Source: three-view drawing plus pictorial views. Frame: mm from the lowest corner of the part. Give positions to 0.01 mm unless a question says otherwise; leave off trailing zeros. Order: outer loops, then holes, each group sorted by start corner. A loop starts at its lowest first (then second) coordinate and runs counter-clockwise, first axis right, second up.
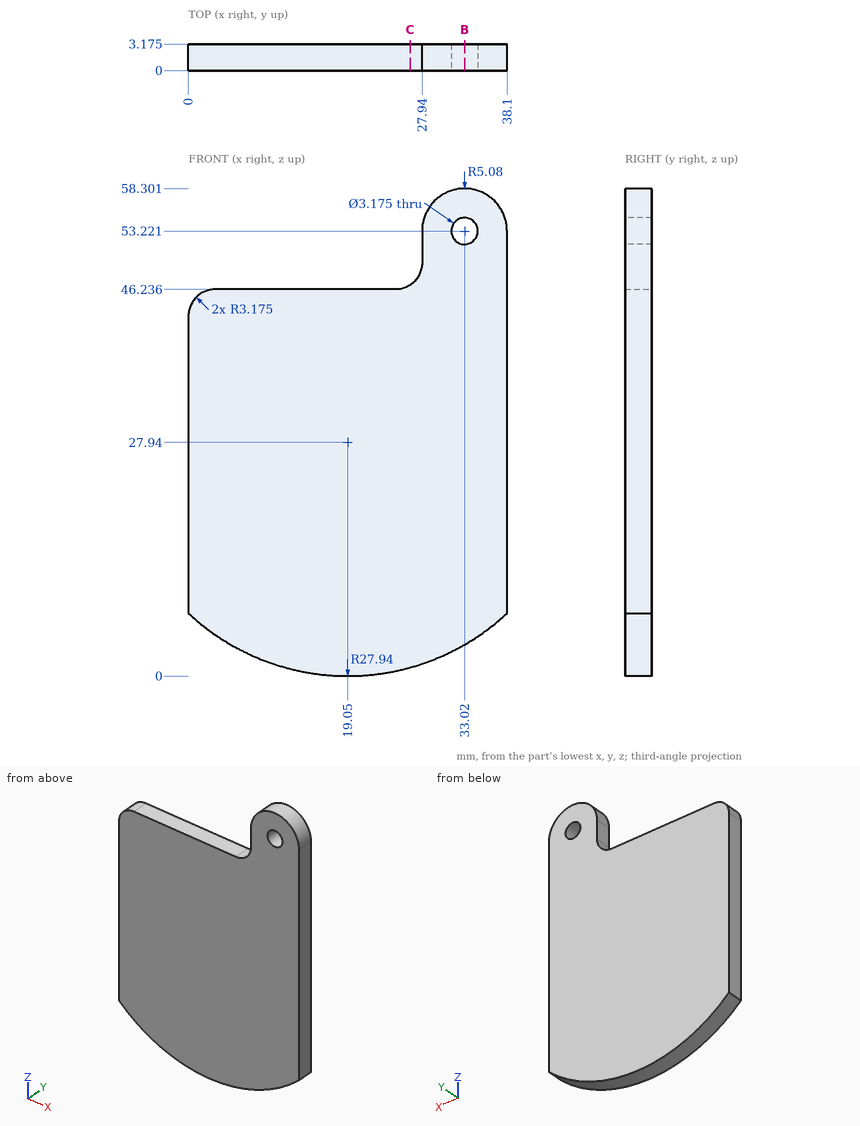
(1) Section B-B, the plane x = 33.02. Return loops of the section in (y, z) (1 decimal), plus the area to 3 significant figures.
(2) Pin query (flat end, axial travel): pin 1 Ø1 at (x, y) = (14.5, 1) entering from +Z; pin 2 Ø1 at (y, z) = (2, 52) entering from -X; pin 3 Ø1.9 at (x, z) = (33.02, 53.22) entering from -Y. Return the tip coordinate at first contact, or that it passes through.
(3) Line query: line 1 along Z through (x, y) = (33.02, 1.5) (1 decimal); line 2 along X through (y, z) = (2, 4) (1 decimal); line 3 along Z through (x, y) = (21, 0.2). Output: solid intervals per line, ascending.
(4) Section C-C, the plane x = 26.5. Return loops of the section in (y, z) (1 decimal), plus the area to 3 significant figures.
Checks:
1. outline: (0, 3.7) - (3.2, 3.7) - (3.2, 51.6) - (0, 51.6) - close; (0, 54.8) - (3.2, 54.8) - (3.2, 58.3) - (0, 58.3) - close
1. area: 163 mm2
2. pin 1: stops at z = 46.24
2. pin 2: stops at x = 27.94
2. pin 3: passes through
3. line 1: z = 3.7 to 51.6, 54.8 to 58.3
3. line 2: x = 4.6 to 33.5
3. line 3: z = 0.07 to 46.24
4. outline: (0, 1) - (3.2, 1) - (3.2, 46.8) - (0, 46.8) - close
4. area: 145 mm2
